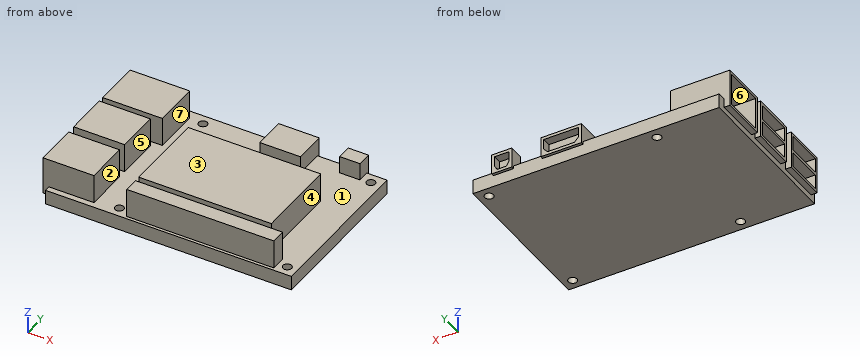
```python
from build123d import *

# Parameters (mm, degrees)
CROQUIS1_W                   = 85
CROQUIS1_H                   = 56
CROQUIS1_R                   = 1.5
SALIENTE_EXTRUIR3_DEPTH      = 5
SALIENTE_EXTRUIR4_DEPTH      = 10
SALIENTE_EXTRUIR4_DEPTH_BACK = 3
CROQUIS2_W                   = 20.6
CROQUIS2_H                   = 16
CROQUIS3_W                   = 50.8
CROQUIS3_H                   = 5.1
SALIENTE_EXTRUIR5_DEPTH      = 10
CROQUIS4_W                   = 11
CROQUIS4_H                   = 14
CORTAR_EXTRUIR2_DEPTH        = 15
CROQUIS5_W                   = 45.8
CROQUIS5_H                   = 28.9
SALIENTE_EXTRUIR6_DEPTH      = 10
SALIENTE_EXTRUIR8_DEPTH      = 10
SALIENTE_EXTRUIR8_DEPTH_BACK = 3
CROQUIS6_W                   = 17.6
CROQUIS6_H                   = 15
CROQUIS7_W                   = 5
CROQUIS7_H                   = 13
CORTAR_EXTRUIR3_DEPTH        = 15
SALIENTE_EXTRUIR9_DEPTH      = 6
SALIENTE_EXTRUIR9_DEPTH_BACK = 1
CROQUIS8_W                   = 7
CROQUIS8_H                   = 5
CROQUIS8_W_2                 = 14
CROQUIS8_H_2                 = 11
CORTAR_EXTRUIR4_DEPTH        = 3


with BuildPart() as part:
    # Croquis1 → Saliente-Extruir3 (new body)
    with BuildSketch(Plane.XY):
        with Locations((42.5, 28)):
            Rectangle(CROQUIS1_W, CROQUIS1_H)
        with Locations((23.5, 52.5)):
            Circle(CROQUIS1_R, mode=Mode.SUBTRACT)
        with Locations((23.5, 3.5)):
            Circle(CROQUIS1_R, mode=Mode.SUBTRACT)
        with Locations((81.5, 52.5)):
            Circle(CROQUIS1_R, mode=Mode.SUBTRACT)
        with Locations((81.5, 3.5)):
            Circle(CROQUIS1_R, mode=Mode.SUBTRACT)
    extrude(amount=SALIENTE_EXTRUIR3_DEPTH)

    # Croquis2 → Saliente-Extruir4 (add, two sides: drawn at the far end of the back side and taken through both)
    with BuildSketch(Plane.XY.offset(5).offset(-SALIENTE_EXTRUIR4_DEPTH_BACK)):
        with Locations((8.3, 45)):
            Rectangle(CROQUIS2_W, CROQUIS2_H)
    extrude(amount=SALIENTE_EXTRUIR4_DEPTH + SALIENTE_EXTRUIR4_DEPTH_BACK)

    # Croquis3 → Saliente-Extruir5 (add)
    with BuildSketch(Plane.XY.offset(5)):
        with Locations((52.9, 3.55)):
            Rectangle(CROQUIS3_W, CROQUIS3_H)
    extrude(amount=SALIENTE_EXTRUIR5_DEPTH)

    # Croquis4 → Cortar-Extruir2 (cut)
    with BuildSketch(Plane.ZY.offset(2)):
        with Locations((8.5, 45)):
            Rectangle(CROQUIS4_W, CROQUIS4_H)
    extrude(amount=-CORTAR_EXTRUIR2_DEPTH, mode=Mode.SUBTRACT)

    # Croquis5 → Saliente-Extruir6 (add)
    with BuildSketch(Plane.XY.offset(5)):
        with Locations((50.4, 22.55)):
            Rectangle(CROQUIS5_W, CROQUIS5_H)
    extrude(amount=SALIENTE_EXTRUIR6_DEPTH)

    # Croquis6 → Saliente-Extruir8 (add, two sides: drawn at the far end of the back side and taken through both)
    with BuildSketch(Plane.XY.offset(5).offset(-SALIENTE_EXTRUIR8_DEPTH_BACK)):
        with Locations((6.8, 27.5)):
            Rectangle(CROQUIS6_W, CROQUIS6_H)
        with Locations((6.8, 9.5)):
            Rectangle(CROQUIS6_W, CROQUIS6_H)
    extrude(amount=SALIENTE_EXTRUIR8_DEPTH + SALIENTE_EXTRUIR8_DEPTH_BACK)

    # Croquis7 → Cortar-Extruir3 (cut)
    with BuildSketch(Plane.ZY.offset(2)):
        with Locations((5.5, 27.5)):
            Rectangle(CROQUIS7_W, CROQUIS7_H)
        with Locations((11.5, 27.5)):
            Rectangle(CROQUIS7_W, CROQUIS7_H)
        with Locations((11.5, 9.5)):
            Rectangle(CROQUIS7_W, CROQUIS7_H)
        with Locations((5.5, 9.5)):
            Rectangle(CROQUIS7_W, CROQUIS7_H)
    extrude(amount=-CORTAR_EXTRUIR3_DEPTH, mode=Mode.SUBTRACT)

    # Croquis8 → Saliente-Extruir9 (add, two sides: drawn at the far end of the back side and taken through both)
    with BuildSketch(Plane.XY.offset(5).offset(-SALIENTE_EXTRUIR9_DEPTH_BACK)):
        with Locations((74.5, 54.5)):
            Rectangle(CROQUIS8_W, CROQUIS8_H)
        with Locations((54, 51.5)):
            Rectangle(CROQUIS8_W_2, CROQUIS8_H_2)
    extrude(amount=SALIENTE_EXTRUIR9_DEPTH + SALIENTE_EXTRUIR9_DEPTH_BACK)

    # Croquis9 → Cortar-Extruir4 (cut)
    with BuildSketch(Plane(origin=(0, 57, 0), x_dir=(1, 0, 0), z_dir=(0, 1, 0))):
        Polygon((48, -10), (60, -10), (60, -6.462110536), (58.635363499, -5), (49.364636501, -5), (48, -6.462110536), align=None)
        Polygon((72, -10), (77, -10), (77, -6.561817621), (76.105167212, -5), (72.894832788, -5), (72, -6.561817621), align=None)
    extrude(amount=-CORTAR_EXTRUIR4_DEPTH, mode=Mode.SUBTRACT)


solid = part.part
```
Here's how the part is built. I have some questions about the finished solid (model axes, mm). Face numbers are marked on the shaded views. A direction names the side the tool comes from. Coordinates: 2 decimals unless noted, no trailing zeros. Order: outer loops, then holes, each group sorted by start corner. A loop starts at its lowest first (then second) coordinate and runs counter-clockwise, first axis right, second up. Notation, with made-up numbers: M 38,89.25 L 56,89.25 A22 ccw 56,101.25 Z; hole C 83.25,49 d10. An arc over 180 degrees is marked long. Answer as a JSON object with one key per item and string values. Group by question number.
(1) Suppose I cut it at D-D, the plane y = 7. Please give me the cut outline in (x, z), then the cut area to 3 significant figures.
(2) Suppose I cut it at C-C, the plane y = 13. Please give me the cut outline in (x, z).
(3) For pin 1 (1.5 mm diameter, centred on x = 4, z = 12.5, fed in from -Y); pin 2 (3 mm diameter, centred on y = 25, z = 12, fed in from +X); pin 3 (1 mm diameter, centred on x = 13, z = 11.5, fed in from +Y), each with a flat end and sliding along its axis, tell me the tip position at first contact or that it passes through.
(4) I need wall thicknesses on probe 1 along Y at (x, z) = (81.5, 2.2); probe 2 along Z at (x, y) = (3, 11.5); probe 3 along Y at (x, z) = (4.5, 7). Which ranges of each line are inside material? Lowest first, please.
(5) Suppose I cut it at A-A, the plane x = 23.5. Please give me the cut outline in (y, z).
(6) Suppose I cut it at B-B, the plane x = 32.5. Please give me the cut outline in (y, z), then the cut area to 3 significant figures.
(7) Which directions (+Z, -Z, +X, -X, +Y, -Y) give clear straight access to the entire face, cutting with the end or side of a thin tool? Please do the marked faces 5, 6 and 7.
(8) If we mould it in two halves opening along X, with no side actions, what happens to the marked faces 1, 2, 3 and 4? For each: released by +X, released by -X, zero draft, split by the parting line, or undercut.
Values found:
{
 "1": {"outline": "M -2,2 L 0,2 L 0,0 L 85,0 L 85,5 L 15.6,5 L 15.6,15 L -2,15 L -2,14 L 13,14 L 13,9 L -2,9 L -2,8 L 13,8 L 13,3 L -2,3 Z", "area": "457 mm^2"},
 "2": {"outline": "M -2,2 L 0,2 L 0,0 L 85,0 L 85,5 L 73.3,5 L 73.3,15 L 27.5,15 L 27.5,5 L 15.6,5 L 15.6,15 L -2,15 L -2,14 L 13,14 L 13,9 L -2,9 L -2,8 L 13,8 L 13,3 L -2,3 Z"},
 "3": {"pin 1": "stops at y = 2", "pin 2": "stops at x = 73.3", "pin 3": "stops at y = 53"},
 "4": {"probe 1": "y = 0 to 2, 5 to 51, 54 to 56", "probe 2": "z = 0 to 3, 8 to 9, 14 to 15", "probe 3": "y = 2 to 3, 16 to 17, 20 to 21, 34 to 35, 37 to 38, 52 to 53"},
 "5": {"outline": "M 0,0 L 2,0 L 2,5 L 0,5 Z; M 5,0 L 51,0 L 51,5 L 5,5 Z; M 54,0 L 56,0 L 56,5 L 54,5 Z"},
 "6": {"outline": "M 0,0 L 56,0 L 56,5 L 37,5 L 37,15 L 8.1,15 L 8.1,5 L 6.1,5 L 6.1,15 L 1,15 L 1,5 L 0,5 Z", "area": "620 mm^2"},
 "7": {"face 5": "+Z, -Y", "face 6": "-X", "face 7": "+Z, +Y, -Y"},
 "8": {"face 1": "undercut", "face 2": "undercut", "face 3": "zero draft", "face 4": "released by +X"}
}
